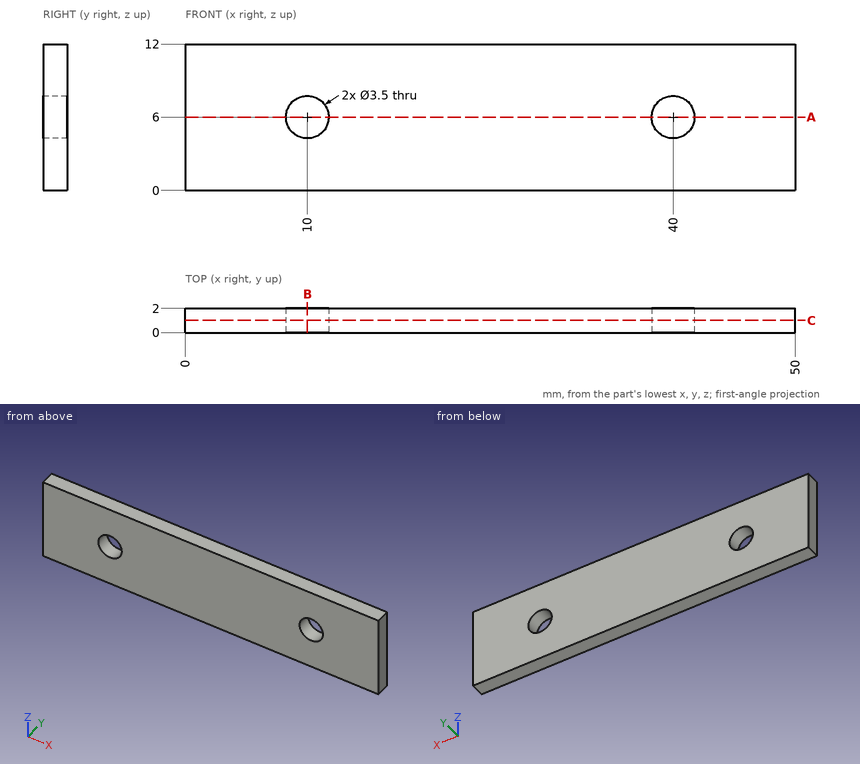
Check sheet for the drawn part. Datum: minimum x, y, z corner. Units: mm. Round coordinates to 2 decimals unless told otherwise and drop trailing zeros. Loops run counter-clockwise (first coordinate to the right, second up) from the corner with the lowest first, then second, coordinate; pieces in that order, holes last. Notation, with made-up numbers: (75, -26) - (133, -26) arc R34 cw to (133, 5) - close; hole circle Ø6 at (19.25, 52.5). An arc over 180 degrees is marked (long way). Write each question's results on one line, items separated by ' | '. Start each with the question number.
Q1. Cross-section at C-C on y = 1. Enter the section's corners in (x, z).
Q2. Cross-section at A-A on z = 6. Enter the section's corners in (x, y), and give its area (3 significant figures).
Q3. Cross-section at B-B on x = 10. Enter the section's corners in (y, z), and give its area (3 significant figures).
Q4. Thickness scan on line 1 (X direction, y = 0.4, z = 6); line 2 (X direction, y = 1.7, z = 5). Record the ranges inside material, lowest first. Write a range as [from, to].
Answers below:
1) outline: (0, 0) - (50, 0) - (50, 12) - (0, 12) - close; hole circle Ø3.5 at (10, 6); hole circle Ø3.5 at (40, 6)
2) outline: (0, 0) - (8.25, 0) - (8.25, 2) - (0, 2) - close; (11.75, 0) - (38.25, 0) - (38.25, 2) - (11.75, 2) - close; (41.75, 0) - (50, 0) - (50, 2) - (41.75, 2) - close | area: 86.0 mm²
3) outline: (0, 0) - (2, 0) - (2, 4.25) - (0, 4.25) - close; (0, 7.75) - (2, 7.75) - (2, 12) - (0, 12) - close | area: 17.0 mm²
4) line 1: x = [0, 8.25], [11.75, 38.25], [41.75, 50] | line 2: x = [0, 8.56], [11.44, 38.56], [41.44, 50]
